Geometry: final body of the model. Coordinates: model frame, mm. A direction names the side the tool comes from. Round coordinates to 2 decimals unless told otherwise and drop trailing zeros. Write each loop counter-clockwise with the first axis right and the second up, starting at its lowest first coordinate (ties: lowest second). Pieces come first, ordered by that corner, then holes. Notation, with made-up numbers: M 8.5,89 L 35.5,89 A32 ccw 35.5,117 Z; hole C 70.5,66 d11. An arc over 180 degrees is marked long. Use one line per item in the form item = value. Start each with the question number.
from build123d import *

# Parameters (mm, degrees)
BOSS_EXTRUDE1_DEPTH   = 32
BOSS_EXTRUDE1_2_DEPTH = 32
BOSS_EXTRUDE2_DEPTH   = 5
BOSS_EXTRUDE3_DEPTH   = 5


with BuildPart() as part:
    # Sketch1 → Boss-Extrude1 (new body)
    with BuildSketch(Plane(origin=(0, 0, 0), x_dir=(-1, 0, 0), z_dir=(0, 0, 1))):
        Polygon((-29.846050857, 76.265916966), (-29.846050857, 79.765916966), (-24.246050857, 79.765916966), (-24.246050857, 85.765916966), (4.753949143, 85.765916966), (4.753949143, 79.765916966), (10.353949143, 79.765916966), (10.353949143, 76.265916966), (15.353949143, 76.265916966), (15.353949143, 84.765916966), (9.753949143, 84.765916966), (9.753949143, 90.765916966), (-29.246050857, 90.765916966), (-29.246050857, 84.765916966), (-34.846050857, 84.765916966), (-34.846050857, 76.265916966), align=None)
    extrude(amount=BOSS_EXTRUDE1_DEPTH)



with BuildPart() as body_2:
    # Sketch1 → Boss-Extrude1 2 (new body)
    with BuildSketch(Plane(origin=(0, 0, 0), x_dir=(-1, 0, 0), z_dir=(0, 0, 1))):
        Polygon((-29.846050857, 50.265916966), (-29.846050857, 45.765916966), (-24.246050857, 45.765916966), (-24.246050857, 39.765916966), (4.753949143, 39.765916966), (4.753949143, 45.765916966), (10.353949143, 45.765916966), (10.353949143, 50.265916966), (15.353949143, 50.265916966), (15.353949143, 40.765916966), (9.753949143, 40.765916966), (9.753949143, 34.765916966), (-29.246050857, 34.765916966), (-29.246050857, 40.765916966), (-34.846050857, 40.765916966), (-34.846050857, 50.265916966), align=None)
    extrude(amount=BOSS_EXTRUDE1_2_DEPTH)


with BuildPart() as part_1:
    add(part.part)

    add(body_2.part)  # Boss-Extrude2 merges body 2
    # Sketch2 → Boss-Extrude2 (add)
    with BuildSketch(Plane.XY.offset(32)):
        Polygon((-9.753949143, -34.765916966), (-9.753949143, -40.765916966), (-15.353949143, -40.765916966), (-15.353949143, -84.765916966), (-9.753949143, -84.765916966), (-9.753949143, -90.765916966), (29.246050857, -90.765916966), (29.246050857, -84.765916966), (34.846050857, -84.765916966), (34.846050857, -40.765916966), (29.246050857, -40.765916966), (29.246050857, -34.765916966), align=None)
    extrude(amount=BOSS_EXTRUDE2_DEPTH)

    # Sketch4 → Boss-Extrude3 (add)
    with BuildSketch(Plane(origin=(0, 0, 0), x_dir=(-1, 0, 0), z_dir=(0, 0, -1))):
        Polygon((-34.846050857, -84.765916966), (-34.846050857, -100.765916966), (15.353949143, -100.765916966), (15.353949143, -84.765916966), (9.753949143, -84.765916966), (9.753949143, -90.765916966), (-29.246050857, -90.765916966), (-29.246050857, -84.765916966), align=None)
    extrude(amount=-BOSS_EXTRUDE3_DEPTH)


solid = part_1.part
1. Contact query for flat-ended pins moving along their axis: pin 1 (4.5 mm diameter, centred on x = -13, z = 11.5, fed in from +Y); pin 2 (6.5 mm diameter, centred on y = -89, z = 28, fed in from -X); pin 3 (2 mm diameter, centred on x = 11.5, z = 17.5, fed in from -Y). Output: stop coordinate, or through.
2. Set-up query: faces 1 (the face through (32, -84.766, 21)), 2 (the face through (-8, -45.766, 16)), 3 (the face through (-9.754, -38, 18)). Return all of +Z, -Z, +X, -X, +Y, -Y with unobstructed straight access to the full face (end or side cutting, diameter ignored); none if empty.
3. Section query D-D (x = 5). Return loops of the section in (y, z), then the cut area to 3 significant figures.
4. Ray query, probe 1 along Y at (x, z) = (21, 19); probe 2 along Y at (x, z) = (-6, 17); probe 3 along X at (y, z) = (-84.5, 17.5). Return the intervals inside material, ascending.
5. Section query B-B (x = -6.5). Return loops of the section in (y, z), then the cut area to 3 significant figures.
6. Section query C-C (y = -47). Return loops of the section in (x, z), then the cut area to 3 significant figures.
7. Pull-direction query (X, two-part tool) for faces 4 (the face through (9, -90.766, 21)), 5 (the face through (34.846, -77, 18)), 6 (the face through (-4.754, -43, 16)), 7 (the face through (24.246, -83, 16)); classes: released by +X, released by -X, zero draft, split by the parting line, or undercut.
Checks:
q1.pin_1 = -40.77
q1.pin_2 = -9.75
q1.pin_3 = -90.77
q2.face_1 = +Z, +X, -Y
q2.face_2 = -Z
q2.face_3 = +Z, -Z, -X, +Y
q3.outline = M -100.77,0 L -85.77,0 L -85.77,32 L -39.77,32 L -39.77,0 L -34.77,0 L -34.77,37 L -90.77,37 L -90.77,5 L -100.77,5 Z
q3.area = 650 mm^2
q4.probe_1 = -90.77 to -85.77, -39.77 to -34.77
q4.probe_2 = -90.77 to -79.77, -45.77 to -34.77
q4.probe_3 = -15.35 to -4.75, 24.25 to 34.85
q5.outline = M -100.77,0 L -79.77,0 L -79.77,32 L -45.77,32 L -45.77,0 L -34.77,0 L -34.77,37 L -90.77,37 L -90.77,5 L -100.77,5 Z
q5.area = 1,030 mm^2
q6.outline = M -15.35,0 L -10.35,0 L -10.35,32 L 29.85,32 L 29.85,0 L 34.85,0 L 34.85,37 L -15.35,37 Z
q6.area = 571 mm^2
q7.face_4 = zero draft
q7.face_5 = released by +X
q7.face_6 = undercut
q7.face_7 = undercut
